The model under review builds one solid part; all positions refer to its coordinate system, in mm. A direction names the side the tool comes from. Give positions to 0.01 mm unless a question says otherwise; leave off trailing zeros. Loops run counter-clockwise (first coordinate to the right, second up) from the corner with the lowest first, then second, coordinate; pieces in that order, holes last. Notation, with made-up numbers: (-12, 39) - (22, 39) arc R34 cw to (22, 77) - close; hole circle Ø3 at (-37, 38.25). An arc over 180 degrees is marked (long way). Return JSON: item names as keys, results as strings. Group by question number.
from build123d import *

# Parameters (mm, degrees)
EXTRUDE_1_DEPTH     = 23
SKETCH_2_R          = 4.25
CUT_EXTRUDE_1_DEPTH = 5
SKETCH_3_R          = 4.25
CUT_EXTRUDE_2_DEPTH = 5
FILLET_1_R          = 4
FILLET_2_R          = 1


with BuildPart() as part:
    # Эскиз1 → Бобышка-Вытянуть1 (new body, symmetric)
    with BuildSketch(Plane.XY):
        Polygon((0, 0), (-42.426406871, 42.426406871), (-38.890872965, 45.961940777), (-15.028558569, 22.099626381), (26.253591352, 5), (60, 5), (60, 0), align=None)
        Polygon((-14.313708499, 18.556349186), (23.242640687, 3), (1.242640687, 3), align=None, mode=Mode.SUBTRACT)
    extrude(amount=EXTRUDE_1_DEPTH, both=True)

    # Эскиз2 → Вырез-Вытянуть1 (cut)
    with BuildSketch(Plane(origin=(0, 0, 0), x_dir=(0, 0, 1), z_dir=(-0.707106781, -0.707106781, 0))):
        with Locations(Location((0, 45, 0), (0, 0, 270))):  # turned: the seam where the file's is
            Circle(SKETCH_2_R)
    extrude(amount=-CUT_EXTRUDE_1_DEPTH, mode=Mode.SUBTRACT)

    # Эскиз3 → Вырез-Вытянуть2 (cut)
    with BuildSketch(Plane.XZ):
        with Locations(Location((45, 0, 0), (0, 0, 270))):  # turned: the seam where the file's is
            Circle(SKETCH_3_R)
    extrude(amount=-CUT_EXTRUDE_2_DEPTH, mode=Mode.SUBTRACT)

    # Скругление1
    fillet_1_edges = [part.edges().sort_by_distance(p)[0] for p in [
        (-38.890872965, 45.961940777, 0),
        (60, 5, 0),
    ]]
    fillet(fillet_1_edges, radius=FILLET_1_R)

    # Скругление2
    fillet_2_edges = [part.edges().sort_by_distance(p)[0] for p in [
        (-14.313708499, 18.556349186, 0),
        (1.242640687, 3, 0),
        (23.242640687, 3, 0),
    ]]
    fillet(fillet_2_edges, radius=FILLET_2_R)


solid = part.part
Item 1: Mouldability with a two-part tool opening along Y and no side actions: class faces 4 (the face through (-38.935, 44.305, -0.322)), 5 (the face through (5, 11, 23)), 6 (the face through (4.27, 10.86, 0.32)) as +Y half, -Y half, draft (parallel to the pull), parting line (faces both ways), or undercut.
Item 2: Take a section at B-B (z = -2.5). State the section outline as (x, y) points.
Item 3: Take a section at C-C (z = -8). State the section outline as (x, y) points, then the cut area to 3 significant figures.
Item 4: For L1, parallel to X at y = 6, z = 0.5; L2, parallel to X at y = 4, z = 16; L3, parallel to Y at x = 4.5, z = -9.5, list the stretches that pass through material, from the lowest coordinate up. Write a range as from..to.
Item 5: Take a section at D-D (x = -1.5). State the section outline as (y, z) points, then the cut area to 3 significant figures.
Item 6: For P1, Ø4, axis at y = 33.5, z = 7, coming from the +X side; P2, Ø2, axis at y = 34, z = -5, coming from the +X side; P3, Ø2, axis at y = 12, z = -1.5, coming from the -X side; P4, Ø7.5, axis at x = 45, z = 0, coming from the +Y side, all flat-tipped, find the tip position at first contact; note any pin that passes through.
Item 7: Take a section at A-A (x = 45). State the section outline as (y, z) points.
Item 8: Tool access review of faces 1 (the face through (40.85, 2.46, 0.92)), 2 (the face through (10, 3, 0)), 3 (the face through (38, 5, 0)): name each direction out of +Z, -Z, +X, -X, +Y, -Y from which nothing blocks a thin tool from reaching the whole face with its end or side.
Check sheet entries:
{
 "1": {"face 4": "+Y half", "face 5": "draft", "face 6": "undercut"},
 "2": {"outline": "(-42.43, 42.43) - (-34.25, 34.25) - (-30.71, 37.79) - (-36.06, 43.13) arc R4 ccw to (-41.72, 43.13) - close; (-29.39, 29.39) - (0, 0) - (41.56, 0) - (41.56, 5) - (26.25, 5) - (-15.03, 22.1) - (-25.85, 32.93) - close; (48.44, 0) - (60, 0) - (60, 1) arc R4 ccw to (56, 5) - (48.44, 5) - close; hole (-10.76, 15) - (0.95, 3.29) arc R1 ccw to (1.66, 3) - (18.22, 3) arc R1 ccw to (18.6, 4.92) - (-9.67, 16.63) arc R1 ccw to start"},
 "3": {"outline": "(-42.43, 42.43) - (0, 0) - (60, 0) - (60, 1) arc R4 ccw to (56, 5) - (26.25, 5) - (-15.03, 22.1) - (-36.06, 43.13) arc R4 ccw to (-41.72, 43.13) - close; hole (-10.76, 15) - (0.95, 3.29) arc R1 ccw to (1.66, 3) - (18.22, 3) arc R1 ccw to (18.6, 4.92) - (-9.67, 16.63) arc R1 ccw to start", "area": "626 mm^2"},
 "4": {"L1": "x = -6..-1.76, 16..23.84", "L2": "x = -4..0.24, 19.22..58.65", "L3": "y = 0..3, 10.76..14.01"},
 "5": {"outline": "(1.5, -23) - (5.74, -23) - (5.74, 23) - (1.5, 23) - close; (13.25, -23) - (16.5, -23) - (16.5, 23) - (13.25, 23) - close", "area": "345 mm^2"},
 "6": {"P1": "stops at x = -24.43", "P2": "stops at x = -25.93", "P3": "stops at x = -13", "P4": "passes through"},
 "7": {"outline": "(0, -23) - (5, -23) - (5, -4.25) - (0, -4.25) - close; (0, 4.25) - (5, 4.25) - (5, 23) - (0, 23) - close"},
 "8": {"face 1": "+Y, -Y", "face 2": "+Z, -Z", "face 3": "+Z, -Z, +X, +Y"}
}
